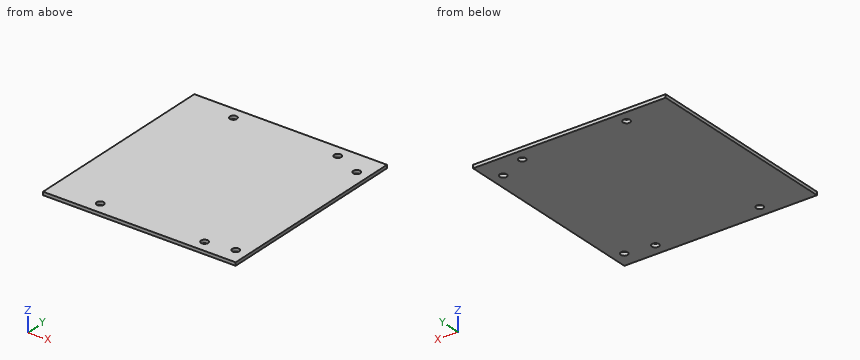
```python
from build123d import *

# Parameters (mm, degrees)
SKETCH_1_W          = 140
SKETCH_1_H          = 125
EXTRUDE_1_DEPTH     = 2
SKETCH_3_R          = 2.2
CUT_EXTRUDE_1_DEPTH = 2
SKETCH_6_R          = 2.2
CUT_EXTRUDE_2_DEPTH = 2
SKETCH_7_R          = 2.2
CUT_EXTRUDE_3_DEPTH = 105
SKETCH_9_W          = 2
SKETCH_9_H          = 125
CUT_EXTRUDE_5_DEPTH = 20


with BuildPart() as part:
    # ｽｹｯﾁ1 → ﾎﾞｽ - 押し出し1 (new body)
    with BuildSketch(Plane.XY):
        Rectangle(SKETCH_1_W, SKETCH_1_H)
    extrude(amount=EXTRUDE_1_DEPTH)

    # ｽｹｯﾁ3 → ｶｯﾄ - 押し出し1 (cut)
    with BuildSketch(Plane.XY.offset(2)):
        with Locations((-60, 58.5)):
            Circle(SKETCH_3_R)
        with Locations((-60, -47.5)):
            Circle(SKETCH_3_R)
    extrude(amount=-CUT_EXTRUDE_1_DEPTH, mode=Mode.SUBTRACT)

    # ｽｹｯﾁ6 → ｶｯﾄ - 押し出し2 (cut)
    with BuildSketch(Plane.XY.offset(2)):
        with Locations((62.5, -52.5)):
            Circle(SKETCH_6_R)
        with Locations((62.5, 47.5)):
            Circle(SKETCH_6_R)
    extrude(amount=-CUT_EXTRUDE_2_DEPTH, mode=Mode.SUBTRACT)

    # ｽｹｯﾁ7 → ｶｯﾄ - 押し出し3 (cut)
    with BuildSketch(Plane.XY.offset(2)):
        with BuildLine():
            ThreePointArc((42.8, 55), (45, 52.8), (47.2, 55))
            Line((47.2, 55), (45, 55))
            Line((45, 55), (42.8, 55))
        make_face()
        with BuildLine():
            Line((45, 55), (47.2, 55))
            ThreePointArc((47.2, 55), (45, 57.2), (42.8, 55))
            Line((42.8, 55), (45, 55))
        make_face()
        with Locations((-20, 55)):
            Circle(SKETCH_7_R)
        with Locations((45, -55)):
            Circle(SKETCH_7_R)
        with Locations((-20, -55)):
            Circle(SKETCH_7_R)
    extrude(amount=-CUT_EXTRUDE_3_DEPTH, mode=Mode.SUBTRACT)

    # ｽｹｯﾁ9 → ｶｯﾄ - 押し出し5 (cut)
    with BuildSketch(Plane.ZY.offset(70)):
        with Locations((1, 0)):
            Rectangle(SKETCH_9_W, SKETCH_9_H)
    extrude(amount=-CUT_EXTRUDE_5_DEPTH, mode=Mode.SUBTRACT)


solid = part.part
```
Model file for the job. Use its own axes, mm. Give positions to 0.01 mm unless a question says otherwise; leave off trailing zeros. Write each loop counter-clockwise with the first axis right and the second up, starting at its lowest first coordinate (ties: lowest second). Pieces come first, ordered by that corner, then holes. Notation, with made-up numbers: (11, 54) -> (24, 54) arc R29 ccw to (24, 87) -> close; hole circle Ø1 at (-18.75, 4.5). An arc over 180 degrees is marked (long way). Use CSV: the item, a comma, the result in double quotes. Start each with the question number.
1) Cut at A-A on y = 47.5. List the corners of the cut face in (x, z).
2) Cut at B-B on x = 45. List the corners of the cut face in (y, z).
3) Pin check, flat tip, straight feed: P1, Ø2.5, axis at x = -20, y = -55, coming from the +Z side. Stop position of the tip, or through.
4) Drill centre lines: L1, parallel to Y at x = 45, z = 1.5; L2, parallel to Y at x = 62.5, z = 1.25. Where is each one in solid material? Low to high.
Final values:
1,outline,"(-50, 0) -> (60.3, 0) -> (60.3, 2) -> (-50, 2) -> close; (64.7, 0) -> (70, 0) -> (70, 2) -> (64.7, 2) -> close"
2,outline,"(-62.5, 0) -> (-57.2, 0) -> (-57.2, 2) -> (-62.5, 2) -> close; (-52.8, 0) -> (52.8, 0) -> (52.8, 2) -> (-52.8, 2) -> close; (57.2, 0) -> (62.5, 0) -> (62.5, 2) -> (57.2, 2) -> close"
3,P1,"passes through"
4,L1,"y = -62.5 to -57.2, -52.8 to 52.8, 57.2 to 62.5"
4,L2,"y = -62.5 to -54.7, -50.3 to 45.3, 49.7 to 62.5"
